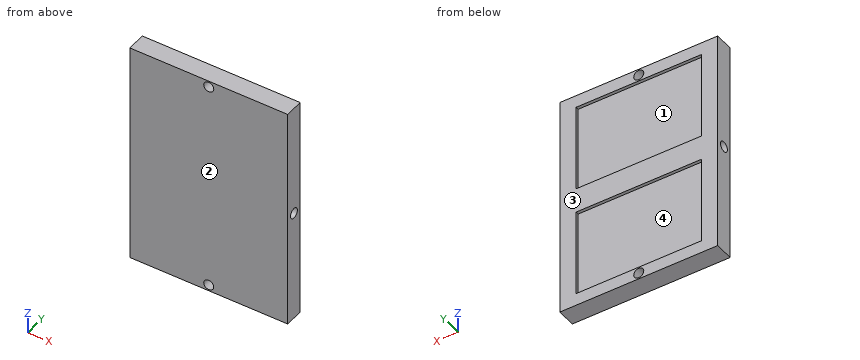
```python
from build123d import *

# Parameters (mm, degrees)
SKETCH1_W               = 126
SKETCH1_H               = 180
BOSS_EXTRUDE1_DEPTH     = 15
SKETCH2_W               = 100
SKETCH2_H               = 70
CUT_EXTRUDE1_DEPTH      = 2.5
SKETCH4_R               = 4
CUT_EXTRUDE3_DEPTH      = 32.5
SKETCH5_R               = 4.1
CUT_EXTRUDE4_DEPTH      = 64
CUT_EXTRUDE4_DEPTH_BACK = 64


with BuildPart() as part:
    # Sketch1 → Boss-Extrude1 (new body)
    with BuildSketch(Plane(origin=(0, 0, 0), x_dir=(1, 0, 0), z_dir=(0, 1, 0))):
        Rectangle(SKETCH1_W, SKETCH1_H)
    extrude(amount=BOSS_EXTRUDE1_DEPTH)

    # Sketch2 → Cut-Extrude1 (cut)
    with BuildSketch(Plane(origin=(0, 15, 0), x_dir=(1, 0, 0), z_dir=(0, 1, 0))):
        with Locations((0, -45)):
            Rectangle(SKETCH2_W, SKETCH2_H)
        with Locations((0, 45)):
            Rectangle(SKETCH2_W, SKETCH2_H)
    extrude(amount=-CUT_EXTRUDE1_DEPTH, mode=Mode.SUBTRACT)

    # Sketch4 → Cut-Extrude3 (cut)
    with BuildSketch(Plane(origin=(0, 0, 0), x_dir=(1, 0, 0), z_dir=(0, 1, 0))):
        with Locations((0, -85)):
            Circle(SKETCH4_R)
        with Locations((0, 85)):
            Circle(SKETCH4_R)
    extrude(amount=CUT_EXTRUDE3_DEPTH, mode=Mode.SUBTRACT)

    # Sketch5 → Cut-Extrude4 (cut, two sides)
    with BuildSketch(Plane(origin=(0, 0, 0), x_dir=(0, 0, -1), z_dir=(1, 0, 0))) as cut_extrude4_sk:
        with Locations((0, 7.5)):
            Circle(SKETCH5_R)
    extrude(amount=CUT_EXTRUDE4_DEPTH, mode=Mode.SUBTRACT)
    extrude(cut_extrude4_sk.sketch, amount=-CUT_EXTRUDE4_DEPTH_BACK, mode=Mode.SUBTRACT)


solid = part.part
```
Geometry check sheet. Reference: the model listing, model coordinates, mm. Face numbers are marked on the shaded views. A direction names the side the tool comes from. Round coordinates to 2 decimals unless told otherwise and drop trailing zeros. Loops run counter-clockwise (first coordinate to the right, second up) from the corner with the lowest first, then second, coordinate; pieces in that order, holes last. Notation, with made-up numbers: (-28.5, 85.5) - (-3.5, 85.5) arc R38 ccw to (-3.5, 123.5) - close; hole circle Ø11 at (55.5, -5.5). An arc over 180 degrees is marked (long way). Write each question's results on one line, items separated by ' | '. Start each with the question number.
Q1. Cross-section at C-C on z = 0. Enter the section's corners in (x, y).
Q2. Release check for a two-part mould opening along Z. For the marked faces 1 and 2 record: +Z half, -Z half, draft (parallel to the pull), parting line (faces both ways), or undercut.
Q3. Gauge pin test, flat end, axial feed: P1, Ø1, axis at x = -35, z = 63.5, coming from the +Y side. Record the tip position at first contact, or that the pin passes through.
Q4. Thickness scan on line 1 (X direction, y = 7, z = -85); line 2 (Z direction, x = -8, y = 8.5); line 3 (Z direction, x = 0, y = 11). Record the ranges inside material, lowest first. Write a range as [from, to].
Q5. Cross-section at A-A on x = 0. Enter the section's corners in (y, z), and give its area (3 significant figures).
Q6. Cross-section at B-B on y = 7.5. Enter the section's corners in (x, z).
Q7. Cross-section at D-D on x = 46. Enter the section's corners in (y, z), and give its area (3 significant figures).
Q8. Access from +Z, -Z, +X, -X, +Y, -Y to the whole of each face (thin tool, end or side, straight path). Record for the marked faces 3 and 4.
Answers below:
1) outline: (-63, 0) - (63, 0) - (63, 3.4) - (-63, 3.4) - close; (-63, 11.6) - (63, 11.6) - (63, 15) - (-63, 15) - close
2) face 1: undercut | face 2: draft
3) P1: stops at y = 12.5
4) line 1: x = [-63, -4], [4, 63] | line 2: z = [-90, -3.98], [3.98, 90] | line 3: z = [-90, -89], [-81, -2.14], [2.14, 81], [89, 90]
5) outline: (0, -90) - (15, -90) - (15, -89) - (0, -89) - close; (0, -81) - (15, -81) - (15, -80) - (12.5, -80) - (12.5, -10) - (15, -10) - (15, 10) - (12.5, 10) - (12.5, 80) - (15, 80) - (15, 81) - (0, 81) - close; (0, 89) - (15, 89) - (15, 90) - (0, 90) - close; hole circle Ø8.2 at (7.5, 0) | area: 2,060 mm²
6) outline: (-63, -90) - (63, -90) - (63, -4.1) - (-63, -4.1) - close; (-63, 4.1) - (63, 4.1) - (63, 90) - (-63, 90) - close; hole circle Ø8 at (0, -85); hole circle Ø8 at (0, 85)
7) outline: (0, -90) - (15, -90) - (15, -80) - (12.5, -80) - (12.5, -10) - (15, -10) - (15, 10) - (12.5, 10) - (12.5, 80) - (15, 80) - (15, 90) - (0, 90) - close; hole circle Ø8.2 at (7.5, 0) | area: 2,300 mm²
8) face 3: +Z, -Z, +X, -X, +Y | face 4: +Y
